Design review of the part built by this model. Coordinates are the model's own, in mm. Give positions to 0.01 mm unless a question says otherwise; leave off trailing zeros. Loops run counter-clockwise (first coordinate to the right, second up) from the corner with the lowest first, then second, coordinate; pieces in that order, holes last. Notation, with made-up numbers: M 69.25,36.5 L 101.25,36.5 A28 ccw 101.25,66.5 Z; hole C 45.25,-24.5 d1. An arc over 180 degrees is marked long. Answer as CSV lines item,"result".
```python
from build123d import *

# Parameters (mm, degrees)
F0_R     = 38.1
F1_DEPTH = 38.1
F3_D     = 34.12998
F4_R     = 6.35


with BuildPart() as f1:
    # F0 (on Front) → F1 (new body, symmetric)
    with BuildSketch(Plane.XZ):
        Circle(F0_R)
    extrude(amount=F1_DEPTH, both=True)

    # F3 (through all)
    with Locations(Plane.XZ.offset(38.1)):
        with Locations((0, 0)):
            Hole(F3_D / 2)

    # F4
    f4_edges = [f1.edges().sort_by_distance(p)[0] for p in [
        (-38.1, -38.1, 0),
        (-38.1, 38.1, 0),
        (-17.06499, 38.1, 0),
        (-17.06499, -38.1, 0),
    ]]
    fillet(f4_edges, radius=F4_R)


solid = f1.part
```
1. We need section A-A, the plane z = 0. Write out the cut boundary in (x, y) (3 decimals), plus the area to 3 significant figures.
Answer block:
outline,"M -38.1,-31.75 A6.35 ccw -31.75,-38.1 L -23.415,-38.1 A6.35 ccw -17.065,-31.75 L -17.065,31.75 A6.35 ccw -23.415,38.1 L -31.75,38.1 A6.35 ccw -38.1,31.75 Z; M 17.065,-31.75 A6.35 ccw 23.415,-38.1 L 31.75,-38.1 A6.35 ccw 38.1,-31.75 L 38.1,31.75 A6.35 ccw 31.75,38.1 L 23.415,38.1 A6.35 ccw 17.065,31.75 Z"
area,"3,140 mm²"
2. For P1, Ø4, axis at x = -28, y = 20, coming from the +Z side; P2, Ø6, axis at x = -12, y = -9, coming from the +Z side; P3, Ø8, axis at x = -15.5, y = 24.5, coming from the -Z side, all flat-tipped, find the tip position at first contact; note any pin that passes through.
Answer block:
P1,"z = 27.85"
P2,"z = 37.02"
P3,"z = -36.32"
3. The part is to be moulded in two halves that separate along Z. For faces 1 (the flat face through (-14, -38.1, -19)), 2 (the cylindrical face through (-30.235, -0.444, -23.183)), 3 (the cylindrical face through (3.7, 0.44, -16.66)), say which applies: pulls with the +Z half, pulls with the -Z half, needs draft (parallel to the pull), parting line crosses it, or undercut.
Answer block:
face 1,"needs draft"
face 2,"parting line crosses it"
face 3,"undercut"
4. We need section C-C, the plane y = -24. Write out the cut boundary in (x, z) (3 decimals), plus the area to 3 significant figures.
Answer block:
outline,"C 0,0 d76.2; hole C 0,0 d34.13"
area,"3,650 mm²"
5. To check wall thickness, follow L1, parallel to Z at x = 0, y = -11.5 (3 decimals); L2, parallel to Y at x = -27.5, z = -16; L3, parallel to X at y = -17.5, z = 7. State the ranges of each line that lie inside material, in increasing order. Write a range as [from, to].
Answer block:
L1,"[-38.1, -17.065], [17.065, 38.1]"
L2,"[-38.1, 38.1]"
L3,"[-37.45, -15.56], [15.56, 37.45]"
6. We need section B-B, the plane x = 0. Write out the cut boundary in (y, z) (3 decimals).
Answer block:
outline,"M -38.1,-31.75 A6.35 ccw -31.75,-38.1 L 31.75,-38.1 A6.35 ccw 38.1,-31.75 L 38.1,-23.415 A6.35 ccw 31.75,-17.065 L -31.75,-17.065 A6.35 ccw -38.1,-23.415 Z; M -38.1,23.415 A6.35 ccw -31.75,17.065 L 31.75,17.065 A6.35 ccw 38.1,23.415 L 38.1,31.75 A6.35 ccw 31.75,38.1 L -31.75,38.1 A6.35 ccw -38.1,31.75 Z"
